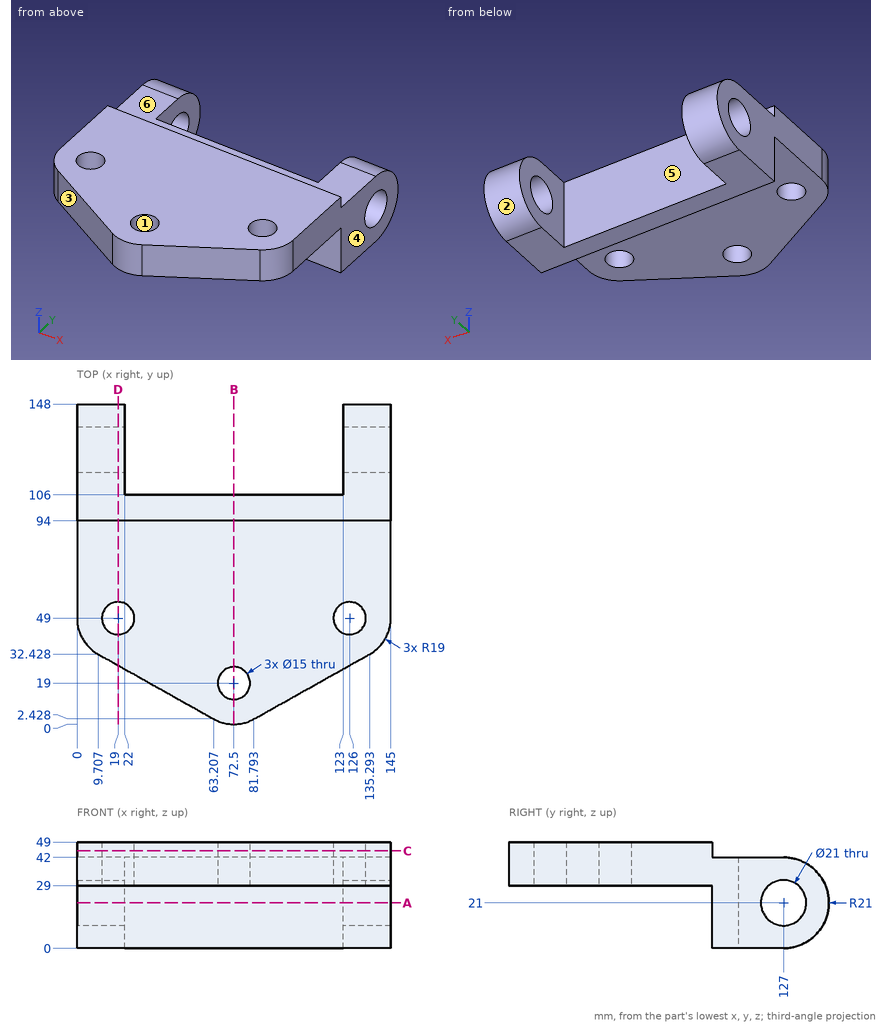
Part print with two shaded views. Sizes in mm from the minimum x, y, z corner. A direction names the side the tool comes from. Coordinates: 2 decimals unless noted, no trailing zeros. Order: outer loops, then holes, each group sorted by start corner. A loop starts at its lowest first (then second) coordinate and runs counter-clockwise, first axis right, second up.
(1) Saw through at D-D, the plane x = 19. Write the cut outline in (y, z).
Solution:
outline: (27.22, 29) - (41.5, 29) - (41.5, 49) - (27.22, 49) - close; (56.5, 29) - (94, 29) - (94, 0) - (127, 0) arc R21 ccw to (127, 42) - (94, 42) - (94, 49) - (56.5, 49) - close; hole circle Ø21 at (127, 21)
(2) Mould opens along Y. For the marked faces 1, 2 and 3 say: released by +Y, released by -Y, zero draft, split by the parting line, or undercut.
Solution:
face 1: undercut
face 2: released by +Y
face 3: released by -Y
(3) Saw through at C-C, the plane z = 45. Write the cut outline in (x, y).
Solution:
outline: (0, 49) arc R19 ccw to (9.71, 32.43) - (63.21, 2.43) arc R19 ccw to (81.79, 2.43) - (135.29, 32.43) arc R19 ccw to (145, 49) - (145, 94) - (0, 94) - close; hole circle Ø15 at (19, 49); hole circle Ø15 at (72.5, 19); hole circle Ø15 at (126, 49)
(4) Pin check, flat tips, straight feed: pin 1 Ø13.5 at (x, y) = (126, 49) entering from +Z; pin 2 Ø1.5 at (x, y) = (86.5, 71) entering from -Z; pin 3 Ø19.5 at (x, y) = (72.5, 19) entering from +Z; pin 4 Ø16.5 at (x, y) = (92.5, 112.5) entering from +Z. Stop position of each tip, or through.
Solution:
pin 1: passes through
pin 2: stops at z = 29
pin 3: stops at z = 49
pin 4: stops at z = 42
(5) Which spindle directions (+Z, -Z, +X, -X, +Y, -Y) get a long thin tool onto all of the face, cutting with end or side? Do the marked faces 4, 5 and 6. Say none if no direction does.
Solution:
face 4: +Z, -Z, +X, +Y, -Y
face 5: +Z, -Z, +Y
face 6: +Z, +X, -X, +Y
(6) Drill centre lines: L1, parallel to X at y = 141.5, z = 17; L2, parallel to Z at x = 7, y = 126.5; L3, parallel to Z at x = 82, y = 34.5. Where is each one in solid material? Low to high.
Solution:
L1: x = 0 to 22, 123 to 145
L2: z = 0 to 10.51, 31.49 to 42
L3: z = 29 to 49
(7) Saw through at B-B, the plane x = 72.5. Write the cut outline in (y, z).
Solution:
outline: (0, 29) - (11.5, 29) - (11.5, 49) - (0, 49) - close; (26.5, 29) - (94, 29) - (94, 0) - (106, 0) - (106, 42) - (94, 42) - (94, 49) - (26.5, 49) - close
(8) Saw through at A-A, the plane z = 21. Write the cut outline in (x, y), and give its area (3 significant figures).
Solution:
outline: (0, 94) - (145, 94) - (145, 116.5) - (123, 116.5) - (123, 106) - (22, 106) - (22, 116.5) - (0, 116.5) - close; (0, 137.5) - (22, 137.5) - (22, 148) - (0, 148) - close; (123, 137.5) - (145, 137.5) - (145, 148) - (123, 148) - close
area: 2,660 mm2
